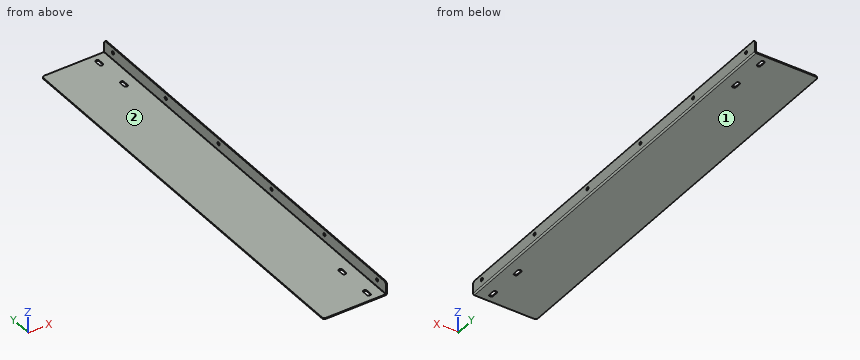
from build123d import *

# Parameters (mm, degrees)
SKETCH_1_W                       = 245
SKETCH_1_H                       = 800
SM_BASE_FLANGE_1_DEPTH           = 2
FILLET_1_R                       = 5
SKETCH_2_W                       = 1
SKETCH_2_H                       = 854.013811654
CUT_EXTRUDE_1_DEPTH              = 10
SKETCH_3_W                       = 130
SKETCH_3_H                       = 800.320249097
CUT_EXTRUDE_2_DEPTH              = 10
SM_EDGE_FLANGE_1_STRIP_W         = 9.4732
SM_EDGE_FLANGE_1_STRIP_H         = 2
SM_EDGE_FLANGE_1_STRIP_CUT_DEPTH = 800
SM_EDGE_FLANGE_1_DEPTH           = 800
FILLET_2_R                       = 5
CUT_EXTRUDE_3_DEPTH              = 10
HOLE_WIZARD_6_0_6_1_D            = 6
PATTERN_LINEAR_1_COUNT           = 6
PATTERN_LINEAR_1_PITCH           = 150


# Sheet-metal steps are written as plain solids
with BuildPart() as part:
    # Sketch 1 → 基体-法兰1 (new body)
    with BuildSketch(Plane.XY):
        Rectangle(SKETCH_1_W, SKETCH_1_H)
    extrude(amount=-SM_BASE_FLANGE_1_DEPTH)

    # 圆角1
    fillet_1_edges = [part.edges().sort_by_distance(p)[0] for p in [
        (-122.5, 400, -1),
        (122.5, 400, -1),
        (122.5, -400, -1),
        (-122.5, -400, -1),
    ]]
    fillet(fillet_1_edges, radius=FILLET_1_R)

    # Sketch 2 → 切除-拉伸1 (cut)
    with BuildSketch(Plane.XY):
        Rectangle(SKETCH_2_W, SKETCH_2_H)
    extrude(amount=-CUT_EXTRUDE_1_DEPTH, mode=Mode.SUBTRACT)


with BuildPart() as cut_extrude_1_piece_1:
    # of the separate pieces the step leaves, piece 1, a body of its own (cut_extrude_1_pieces)
    add(part.part.solids().sort_by_distance((-0.5, -400, 0))[0])

    # 边线-法兰1 strip (across the edge) → 边线-法兰1 strip cut (cut)
    with BuildSketch(Plane(origin=(-0.5, -400, 0), x_dir=(-1, 0, 0), z_dir=(0, 1, 0))):
        with Locations((-2, -1)):
            Rectangle(SM_EDGE_FLANGE_1_STRIP_W, SM_EDGE_FLANGE_1_STRIP_H)
    extrude(amount=SM_EDGE_FLANGE_1_STRIP_CUT_DEPTH, mode=Mode.SUBTRACT)

    # 边线-法兰1 section (across the edge) → 边线-法兰1 (add)
    with BuildSketch(Plane(origin=(-0.5, -400, 0), x_dir=(-1, 0, 0), z_dir=(0, 1, 0))):
        with BuildLine():
            Line((0, 0.7366), (0, 23))
            Line((0, 23), (2, 23))
            Line((2, 23), (2, 0.7366))
            ThreePointArc((2, 0.7366), (2.215745145, 0.215745145), (2.7366, 0))
            Line((2.7366, 0), (2.7366, -2))
            ThreePointArc((2.7366, -2), (0.801531583, -1.198468417), (0, 0.7366))
        make_face()
    extrude(amount=SM_EDGE_FLANGE_1_DEPTH)

    # 圆角2
    fillet_2_edges = [cut_extrude_1_piece_1.edges().sort_by_distance(p)[0] for p in [
        (-1.5, -400, 23),
        (-1.5, 400, 23),
    ]]
    fillet(fillet_2_edges, radius=FILLET_2_R)

    # 草图9 → 切除-拉伸3 (cut)
    with BuildSketch(Plane.XY):
        with BuildLine():
            Line((-22, 385), (-22, 375))
            ThreePointArc((-22, 375), (-25.5, 371.5), (-29, 375))
            Line((-29, 375), (-29, 385))
            ThreePointArc((-29, 385), (-25.5, 388.5), (-22, 385))
        make_face()
        with BuildLine():
            Line((-22, 315), (-22, 305))
            ThreePointArc((-22, 305), (-25.5, 301.5), (-29, 305))
            Line((-29, 305), (-29, 315))
            ThreePointArc((-29, 315), (-25.5, 318.5), (-22, 315))
        make_face()
        with BuildLine():
            Line((-29, -385), (-29, -375))
            ThreePointArc((-29, -375), (-25.5, -371.5), (-22, -375))
            Line((-22, -375), (-22, -385))
            ThreePointArc((-22, -385), (-25.5, -388.5), (-29, -385))
        make_face()
        with BuildLine():
            Line((-22, -305), (-22, -315))
            ThreePointArc((-22, -315), (-25.5, -318.5), (-29, -315))
            Line((-29, -315), (-29, -305))
            ThreePointArc((-29, -305), (-25.5, -301.5), (-22, -305))
        make_face()
    extrude(amount=-CUT_EXTRUDE_3_DEPTH, mode=Mode.SUBTRACT)

    # Ø6.0 (6) 直径孔1 (through all)
    with Locations(Plane.ZY.offset(2.5)):
        with Locations((13, 375)):
            hole_wizard_6_0_6_1 = Hole(HOLE_WIZARD_6_0_6_1_D / 2)

    # 阵列(线性)1: Ø6.0 (6) 直径孔1 ×6
    with Locations(*[(0, -i * PATTERN_LINEAR_1_PITCH, 0) for i in range(1, PATTERN_LINEAR_1_COUNT)]):
        add(hole_wizard_6_0_6_1, mode=Mode.SUBTRACT)


with BuildPart() as cut_extrude_1_piece_2:
    # of the separate pieces the step leaves, piece 2, a body of its own (cut_extrude_1_pieces)
    add(part.part.solids().sort_by_distance((117.5, -400, 0))[0])

    # Sketch 3 → 切除-拉伸2 (cut)
    with BuildSketch(Plane.XY):
        with Locations((65.5, -0.160124549)):
            Rectangle(SKETCH_3_W, SKETCH_3_H)
    extrude(amount=-CUT_EXTRUDE_2_DEPTH, mode=Mode.SUBTRACT)


solid = cut_extrude_1_piece_1.part
Model file for the job. Use its own axes, mm. Face numbers are marked on the shaded views. A direction names the side the tool comes from. Give positions to 0.01 mm unless a question says otherwise; leave off trailing zeros. Order: outer loops, then holes, each group sorted by start corner. A loop starts at its lowest first (then second) coordinate and runs counter-clockwise, first axis right, second up. Notation, with made-up numbers: M 21.25,31 L 79.25,31 A24 ccw 79.25,48 Z; hole C -6,44 d2. An arc over 180 degrees is marked long. Put each result on its own line as item: value. Start each with the question number.
(1) Pin check, flat tips, straight feed: pin 1 Ø1 at (y, z) = (311, -0.5) entering from +X; pin 2 Ø2 at (y, z) = (-379.5, -1.5) entering from +X; pin 3 Ø1 at (y, z) = (184, 1) entering from -X. Stop position of each tip, or through.
(2) Drill centre lines: L1, parallel to X at y = -154, z = 2; L2, parallel to Z at x = -18, y = -217; L3, parallel to Z at x = -2, y = 375. Where is each one in solid material? Low to high. Write a range as [from, to].
(3) Tool access for the marked faces 1 and 2: list every direction of +Z, -Z, +X, -X, +Y, -Y with a clear straight run to the whole face (end or side of a thin tool).
(4) Band-saw the part on A-A on y = -107.5. Give the cut face in (x, z).
(5) Band-saw the part on B-B on x = -103.5. Give the cut face in (y, z), then the cut area to 3 significant figures.
Results below:
1. pin 1: stops at x = -0.6
1. pin 2: stops at x = -0.8
1. pin 3: stops at x = -2.54
2. L1: x = [-2.5, -0.5]
2. L2: z = [-2, 0]
2. L3: z = [-1.7, 10], [16, 23]
3. face 1: -Z, +X, -X, +Y, -Y
3. face 2: +Z, -X, +Y, -Y
4. outline: M -122.5,-2 L -3.24,-2 A2.74 ccw -0.5,0.74 L -0.5,23 L -2.5,23 L -2.5,0.74 A0.74 cw -3.24,0 L -122.5,0 Z
5. outline: M -400,-2 L 400,-2 L 400,0 L -400,0 Z
5. area: 1,600 mm2
